Input: part model. Units: mm. Frame: model coordinates. A direction names the side the tool comes from. Coordinates: 2 decimals unless noted, no trailing zeros. Write each loop counter-clockwise with the first axis right and the second up, starting at its lowest first coordinate (ties: lowest second). Pieces come first, ordered by that corner, then holes. Notation, with made-up numbers: M 34,17.5 L 61,17.5 A26 cw 61,33.5 Z; hole C 85,-24 d1. An arc over 180 degrees is marked long. Use CSV: the item, a comma, the result in double quotes.
Autodesk Inventor part; units mm, degrees
ref_plane "YZ Plane" through (0, 0, 0) normal (1, 0, 0) x (0, 1, 0)
ref_plane "XZ Plane" through (0, 0, 0) normal (0, 1, 0) x (-1, 0, 0)
ref_plane "XY Plane" through (0, 0, 0) normal (0, 0, 1) x (1, 0, 0)
sketch "Sketch1" plane through (0, 0, 0) normal (0, 0, 1) x (1, 0, 0)
  circle A0 centre (0, 0) radius 38.1
  dimension "d0" = 76.2
extrude "Extrusion1" add sketch "Sketch1" along normal blind 25.4
sketch "Sketch2" plane through (0, 0, 25.4) normal (0, 0, 1) x (1, 0, 0)
  circle A0 centre (0, 0) radius 38.1
  circle A1 centre (0, 0) radius 12.7
  dimension "d3" = 25.4
extrude "Extrusion2" cut sketch "Sketch2" against normal blind 2.54 contours A1
sketch "Sketch3" plane through (0, 0, 0) normal (0, 0, -1) x (-1, 0, 0)
  circle A0 centre (0, 0) radius 38.1
  circle A1 centre (0, 0) radius 12.7
  dimension "d6" = 25.4
extrude "Extrusion3" cut sketch "Sketch3" against normal blind 2.54 contours A1
fillet "Fillet1" radius 3.175 2 edges at (-38.1, 0, 25.4) (-38.1, 0, 0)
sketch "Sketch4" plane through (0, 0, 22.86) normal (0, 0, 1) x (1, 0, 0)
  circle A0 centre (0, 0) radius 12.7
  circle A1 centre (0, 0) radius 6.35
  dimension "d10" = 12.7
extrude "Extrusion4" add sketch "Sketch4" along normal blind 6.35 contours A1
sketch "Sketch5" plane through (0, 0, 2.54) normal (0, 0, -1) x (-1, 0, 0)
  circle A0 centre (0, 0) radius 12.7
  circle A1 centre (0, 0) radius 6.35
  dimension "d13" = 12.7
extrude "Extrusion5" add sketch "Sketch5" along normal blind 6.35 contours A1
properties part number "rubber wheel"
1. Contact query for flat-ended pins moving along their axis: pin 1 Ø10 at (x, z) = (1.5, 13.5) entering from -Y; pin 2 Ø5 at (x, z) = (-3, 5.5) entering from +Y; pin 3 Ø12 at (y, z) = (8, 2) entering from -X. Output: stop coordinate, or through.
Resolved:
pin 1,"stops at y = -38.1"
pin 2,"stops at y = 38.1"
pin 3,"stops at x = -38.04"
2. Mould query, pull axis X, two halves, no side actions, for faces 4 (the cylindrical face through (-30.235, 23.183, 12.567)), 5 (the cylindrical face through (-1.38, 6.2, 25.99)), 6 (the flat face through (0, -15, 25.4)). Classes: pulls with the +X half, pulls with the -X half, needs draft (parallel to the pull), parting line crosses it, or undercut.
Resolved:
face 4,"parting line crosses it"
face 5,"undercut"
face 6,"needs draft"
3. Material intervals for line 1 (Y direction, x = 0, z = 0.65); line 2 (Y direction, x = 0, z = 1.3); line 3 (Z direction, x = 29, y = -10), sorted ascending. Write a range as [from, to].
Resolved:
line 1,"y = [-36.85, -12.7], [-6.35, 6.35], [12.7, 36.85]"
line 2,"y = [-37.49, -12.7], [-6.35, 6.35], [12.7, 37.49]"
line 3,"z = [0, 25.4]"
4. Section C-C (z = 20). Return loops of the section in (x, y).
Resolved:
outline,"C 0,0 d76.2"
5. Section A-A (y = 0). Return loops of the section in (x, z) (3 decimals), then the cut area to 3 significant figures.
Resolved:
outline,"M -38.1,3.175 A3.175 ccw -34.925,0 L -12.7,0 L -12.7,2.54 L -6.35,2.54 L -6.35,-3.81 L 6.35,-3.81 L 6.35,2.54 L 12.7,2.54 L 12.7,0 L 34.925,0 A3.175 ccw 38.1,3.175 L 38.1,22.225 A3.175 ccw 34.925,25.4 L 12.7,25.4 L 12.7,22.86 L 6.35,22.86 L 6.35,29.21 L -6.35,29.21 L -6.35,22.86 L -12.7,22.86 L -12.7,25.4 L -34.925,25.4 A3.175 ccw -38.1,22.225 Z"
area,"1,960 mm^2"
6. Access query for faces 1 (the cylindrical face through (-2.75, -12.4, 24.15)), 2 (the flat face through (-3, 6, 2.54)), 3 (the flat face through (0, 0, 29.21)). Directions: +Z, -Z, +X, -X, +Y, -Y. A direction counts if a zero-diameter tool reaches every point of the face in a straight line with its end or side. Return the directions, or none.
Resolved:
face 1,"+Z"
face 2,"-Z"
face 3,"+Z, +X, -X, +Y, -Y"
